For this review, take the finished solid that the model builds, in its own axes (mm). Face numbers are marked on the shaded views. A direction names the side the tool comes from. Give positions to 0.01 mm unless a question says otherwise; leave off trailing zeros. Write each loop counter-clockwise with the first axis right and the second up, starting at its lowest first coordinate (ties: lowest second). Pieces come first, ordered by that corner, then holes.
1) We need section B-B on y = 0. Give the boundary of the cut face in (x, z).
2) Machinability: for the marked faces 4, 5 and 6, which of the approach directions +Z, -Z, +X, -X, +Y, -Y give a long, thin tool a straight path to every point of the face, cutting with its end or side? Answer none if there is none.
3) We need section C-C on z = -9. Give the boundary of the cut face in (x, y), and give its area (3 significant figures).
4) Wall thickness on line 1 along Z through (x, y) = (1.45, 0); line 2 along Z through (x, y) = (-0.15, 1); line 3 along X through (y, z) = (7.5, -4): over which ranges is each line inside the solid? List them lowest first.
5) Draft analysis for pull direction Y (two halves, no side actions). For the marked faces 1, 2 and 3, state which applies: pulls with the +Y half, pulls with the -Y half, needs draft (parallel to the pull), parting line crosses it, or undercut.
6) We need section A-A on x = -0.7. Give the boundary of the cut face in (y, z), and give its area (3 significant figures).
7) For P1, Ø1.7, axis at x = -0.5, y = 1, coming from the -Z side; P2, Ø1, axis at x = 0.5, y = -9, coming from the +Z side; P3, Ø1, axis at x = -1, y = 3, coming from the +Z side; P4, Ø1.3, axis at y = 0, z = -9, coming from the -X side, all flat-tipped, find the tip position at first contact; note any pin that passes through.
8) We need section D-D on z = 0. Give the boundary of the cut face in (x, y), and give its area (3 significant figures).
from build123d import *

# Parameters (mm, degrees)
F0_R     = 11.5
F0_R_2   = 1.05
F1_DEPTH = 2
F2_W     = 8.8
F2_H     = 8.8
F3_DEPTH = 2.1


with BuildPart() as f1:
    # F0 (on Right) → F1 (new body)
    with BuildSketch(Plane.YZ):
        Circle(F0_R)
        with Locations((0, -9)):
            Circle(F0_R_2, mode=Mode.SUBTRACT)
        with Locations((0, 9)):
            Circle(F0_R_2, mode=Mode.SUBTRACT)
    extrude(amount=F1_DEPTH)

    # F2 (on face) → F3 (join)
    with BuildSketch(Plane(origin=(0, 0, 0), x_dir=(0, -1, 0), z_dir=(-1, 0, 0))):
        Rectangle(F2_W, F2_H)
        with BuildLine():
            ThreePointArc((-3, 2), (-2.707107, 2.707107), (-2, 3))
            Line((-2, 3), (2, 3))
            ThreePointArc((2, 3), (2.707107, 2.707107), (3, 2))
            Line((3, 2), (3, -2))
            ThreePointArc((3, -2), (2.707107, -2.707107), (2, -3))
            Line((2, -3), (-2, -3))
            ThreePointArc((-2, -3), (-2.707107, -2.707107), (-3, -2))
            Line((-3, -2), (-3, 2))
        make_face(mode=Mode.SUBTRACT)
    extrude(amount=F3_DEPTH)


solid = f1.part
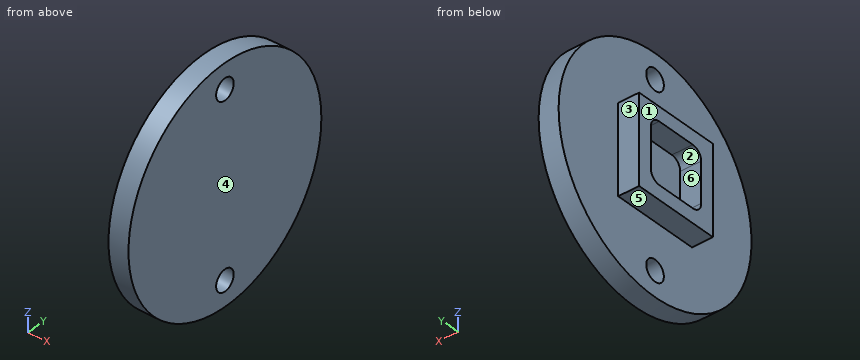
Results list:
1. outline: (-2.1, -4.4) - (0, -4.4) - (0, -7.95) - (2, -7.95) - (2, 7.95) - (0, 7.95) - (0, 4.4) - (-2.1, 4.4) - (-2.1, 3) - (0, 3) - (0, -3) - (-2.1, -3) - close; (0, -11.5) - (2, -11.5) - (2, -10.05) - (0, -10.05) - close; (0, 10.05) - (2, 10.05) - (2, 11.5) - (0, 11.5) - close
2. face 4: +Z, -Z, +X, +Y, -Y
2. face 5: -Z, -X, +Y, -Y
2. face 6: -X
3. outline: (0, -7.16) - (2, -7.16) - (2, -1.05) - (0, -1.05) - close; (0, 1.05) - (2, 1.05) - (2, 7.16) - (0, 7.16) - close
3. area: 24.4 mm2
4. line 1: z = -11.5 to -10.05, -7.95 to 7.95, 10.05 to 11.5
4. line 2: z = -4.4 to -3, 3 to 4.4
4. line 3: x = 0 to 2
5. face 1: needs draft
5. face 2: undercut
5. face 3: pulls with the +Y half
6. outline: (-4.4, -4.4) - (4.4, -4.4) - (4.4, 4.4) - (-4.4, 4.4) - close; hole (-3, -2) arc R1 ccw to (-2, -3) - (2, -3) arc R1 ccw to (3, -2) - (3, 2) arc R1 ccw to (2, 3) - (-2, 3) arc R1 ccw to (-3, 2) - close
6. area: 42.3 mm2
7. P1: stops at z = -11.5
7. P2: stops at z = 7.75
7. P3: stops at z = 4.4
7. P4: passes through
8. outline: (-2.1, -4.4) - (0, -4.4) - (0, -11.5) - (2, -11.5) - (2, 11.5) - (0, 11.5) - (0, 4.4) - (-2.1, 4.4) - (-2.1, 3) - (0, 3) - (0, -3) - (-2.1, -3) - close
8. area: 51.9 mm2
